Check sheet for the modelled part. Datum: model origin and axes. Units: mm. A direction names the side the tool comes from. Round coordinates to 2 decimals unless told otherwise and drop trailing zeros. Order: outer loops, then holes, each group sorted by start corner. A loop starts at its lowest first (then second) coordinate and runs counter-clockwise, first axis right, second up. Notation, with made-up numbers: M 43.5,25.5 L 98.5,25.5 A13 cw 98.5,49.5 Z; hole C 22.5,25.25 d6. An arc over 180 degrees is marked long. One line per item, written item: value. Start each with the question number.
(1) Thickness scan on L1, parallel to Y at x = 160.02, z = 13.25; L2, parallel to Y at x = 126.5, z = 30.5; L3, parallel to Z at x = 210.5, y = 43.5. Record the ranges inside material, lowest first.
(2) Depth check by flat-ended pin: pin 1 Ø15 at (y, z) = (-131.5, -23) entering from -X; pin 2 Ø3 at (x, y) = (207, -129) entering from -Z; pin 3 Ø1.5 at (y, z) = (-105.5, 18) entering from -X; pin 4 Ø4.5 at (x, y) = (213.5, -122) entering from +Z. Enter the tip coordinate at first touch or a pass-through.
(3) Cross-section at B-B, the plane y = -83.5. Enter the section's corners in (x, z), and give its area (3 significant figures).
(4) Access from +Z, -Z, +X, -X, +Y, -Y to the whole of each face (thin tool, end or side, straight path). Record for faces 1 (the face through (158, 124.617, 25)), 2 (the face through (161, -72, 25.4)), 3 (the face through (215, -124, 28.566)), 4 (the face through (162, -142.672, 5)), 5 (the face through (210, 120, -13.97)).
(5) Release check for a two-part mould opening along Y. For faces 6 (the face through (163, 130.967, 6)), 7 (the face through (122, -139, 55.88)), 8 (the face through (212.547, 116, -21)), 9 (the face through (160, 61, 27.94)) record: released by +Y, released by -Y, zero draft, split by the parting line, or undercut.
(6) Cross-section at D-D, the plane z = -36. Enter the section's corners in (x, y).
(7) Cross-section at A-A, the plane z = 12.5. Enter the section's corners in (x, y) (3 decimals), and give its area (3 significant figures).
(8) Cross-section at C-C, the plane z = -8. Enter the section's corners in (x, y).
from build123d import *

# Parameters (mm, degrees)
SKETCH7_R                = 36.83
SKETCH7_R_2              = 1.905
BOSS_EXTRUDE1_DEPTH      = 6.35
SKETCH8_R                = 36.83
BOSS_EXTRUDE2_DEPTH      = 25.4
BOSS_EXTRUDE2_DEPTH_BACK = 0.000254
SKETCH9_R                = 34.925
CUT_EXTRUDE4_DEPTH       = 25.4
BOSS_EXTRUDE3_DEPTH      = 3.175
BOSS_EXTRUDE4_DEPTH      = 38.1
BOSS_EXTRUDE4_DEPTH_BACK = 40.64
CUT_EXTRUDE5_START       = -20.32
SKETCH12_W               = 34.495809925
SKETCH12_H               = 261.703089784
CUT_EXTRUDE5_DEPTH       = 48.26
SKETCH18_W               = 80.102069995
SKETCH18_H               = 6.35
SKETCH18_W_2             = 84.52860838
BOSS_EXTRUDE7_DEPTH      = 66.04
BOSS_EXTRUDE7_DEPTH_BACK = 55.88
MAIN_ANGLE_DEPTH         = 274.638700862
SKETCH19_W               = 12.7
SKETCH19_H               = 12.7
CUT_EXTRUDE8_DEPTH       = 45.72
SKETCH20_W               = 18.203212612
SKETCH20_H               = 62.726676146
CUT_EXTRUDE9_DEPTH       = 6.35
CUT_EXTRUDE9_TAPER       = 26
SKETCH23_R               = 1.905
CUT_EXTRUDE10_DEPTH      = 56.88
SKETCH24_W               = 16.196066748
SKETCH24_H               = 62.242020171
BOSS_EXTRUDE10_DEPTH     = 3.81


with BuildPart() as part:
    # Sketch7 → Boss-Extrude1 (new body)
    with BuildSketch(Plane.XY):
        with BuildLine():
            Line((117.378076693, -136.321789995), (117.378076693, 124.616910866))
            Line((117.378076693, 124.616910866), (117.378076693, 130.966910866))
            Line((117.378076693, 130.966910866), (187.228076693, 130.966910866))
            ThreePointArc((187.228076693, 130.966910866), (205.188588935, 123.527423108), (212.628076693, 105.566910866))
            Line((212.628076693, 105.566910866), (212.628076693, -117.271789995))
            ThreePointArc((212.628076693, -117.271789995), (205.188588935, -135.232302238), (187.228076693, -142.671789995))
            Line((187.228076693, -142.671789995), (117.378076693, -142.671789995))
            Line((117.378076693, -142.671789995), (117.378076693, -136.321789995))
        make_face()
        with Locations((159.923076693, 61.116910866)):
            Circle(SKETCH7_R, mode=Mode.SUBTRACT)
        with Locations((159.923076693, -72.821789995)):
            Circle(SKETCH7_R, mode=Mode.SUBTRACT)
        with Locations((198.520756421, 117.007578537)):
            Circle(SKETCH7_R_2, mode=Mode.SUBTRACT)
        with Locations((198.520756421, -128.598951794)):
            Circle(SKETCH7_R_2, mode=Mode.SUBTRACT)
    extrude(amount=BOSS_EXTRUDE1_DEPTH)

    # Sketch8 → Boss-Extrude2 (add, two sides)
    with BuildSketch(Plane.XY.offset(2.54)) as boss_extrude2_sk:
        with Locations((160.02, 60.978458264)):
            Circle(SKETCH8_R)
        with Locations((160.02, -72.960242597)):
            Circle(SKETCH8_R)
    extrude(amount=BOSS_EXTRUDE2_DEPTH)
    extrude(boss_extrude2_sk.sketch, amount=-BOSS_EXTRUDE2_DEPTH_BACK)

    # Sketch9 → Cut-Extrude4 (cut)
    with BuildSketch(Plane(origin=(0, 0, 0), x_dir=(-1, 0, 0), z_dir=(0, 0, -1))):
        with Locations((-160.02, 60.978458264)):
            Circle(SKETCH9_R)
        with Locations((-160.02, -72.960242597)):
            Circle(SKETCH9_R)
    extrude(amount=-CUT_EXTRUDE4_DEPTH, mode=Mode.SUBTRACT)

    # Sketch10 → Boss-Extrude3 (add)
    with BuildSketch(Plane.XY.offset(6.35)):
        with BuildLine():
            Line((187.228076693, 130.966910866), (187.228076693, 105.566910866))
            Line((187.228076693, 105.566910866), (212.628076693, 105.566910866))
            ThreePointArc((212.628076693, 105.566910866), (205.188588935, 123.527423108), (187.228076693, 130.966910866))
        make_face()
        with BuildLine():
            Line((212.628076693, -117.271789995), (187.228076693, -117.271789995))
            Line((187.228076693, -117.271789995), (187.228076693, -142.671789995))
            ThreePointArc((187.228076693, -142.671789995), (205.188588935, -135.232302238), (212.628076693, -117.271789995))
        make_face()
    extrude(amount=-BOSS_EXTRUDE3_DEPTH)

    # Sketch11 → Boss-Extrude4 (add, two sides)
    with BuildSketch(Plane(origin=(0, 0, 0), x_dir=(-1, 0, 0), z_dir=(0, 0, -1))) as boss_extrude4_sk:
        with BuildLine():
            Line((-217.892216682, -132.511789995), (-217.892216682, 120.806910866))
            ThreePointArc((-217.892216682, 120.806910866), (-214.916421579, 127.991115763), (-207.732216682, 130.966910866))
            Line((-207.732216682, 130.966910866), (-187.228076693, 130.966910866))
            ThreePointArc((-187.228076693, 130.966910866), (-205.188588935, 123.527423108), (-212.628076693, 105.566910866))
            Line((-212.628076693, 105.566910866), (-212.628076693, -117.271789995))
            ThreePointArc((-212.628076693, -117.271789995), (-205.188588935, -135.232302238), (-187.228076693, -142.671789995))
            Line((-187.228076693, -142.671789995), (-207.732216682, -142.671789995))
            ThreePointArc((-207.732216682, -142.671789995), (-214.916421579, -139.695994892), (-217.892216682, -132.511789995))
        make_face()
    extrude(amount=BOSS_EXTRUDE4_DEPTH)
    extrude(boss_extrude4_sk.sketch, amount=-BOSS_EXTRUDE4_DEPTH_BACK)

    # Sketch12 → Cut-Extrude5 (cut)
    with BuildSketch(Plane.XY.offset(6.35).offset(CUT_EXTRUDE5_START)):
        with Locations((195.299001462, -6.234634026)):
            Rectangle(SKETCH12_W, SKETCH12_H)
    extrude(amount=-CUT_EXTRUDE5_DEPTH, mode=Mode.SUBTRACT)

    # Sketch18 → Boss-Extrude7 (add, two sides)
    with BuildSketch(Plane(origin=(0, 0, 0), x_dir=(-1, 0, 0), z_dir=(0, 0, -1))) as boss_extrude7_sk:
        with Locations((-157.429111691, 127.791910866)):
            Rectangle(SKETCH18_W, SKETCH18_H)
        with Locations((-159.642380883, -139.496789995)):
            Rectangle(SKETCH18_W_2, SKETCH18_H)
    extrude(amount=BOSS_EXTRUDE7_DEPTH)
    extrude(boss_extrude7_sk.sketch, amount=-BOSS_EXTRUDE7_DEPTH_BACK)

    # Sketch16 → main angle (cut, through all)
    with BuildSketch(Plane(origin=(0, 130.966910866, 0), x_dir=(1, 0, 0), z_dir=(0, 1, 0))):
        Polygon((217.892216682, 26.67), (-101.016881875, 82.73406518), (217.892216682, 82.73406518), align=None)
        Polygon((217.892216682, -32.396277701), (47.589100189, -76.347646381), (217.892216682, -67.47666805), align=None)
    extrude(amount=-MAIN_ANGLE_DEPTH, mode=Mode.SUBTRACT)

    # Sketch19 → Cut-Extrude8 (cut)
    with BuildSketch(Plane(origin=(217.892216682, 0, 0), x_dir=(0, 0, -1), z_dir=(1, 0, 0))):
        with Locations((-22.215809399, -123.786574298)):
            Rectangle(SKETCH19_W, SKETCH19_H)
        with Locations((-22.215809399, 114.456910866)):
            Rectangle(SKETCH19_W, SKETCH19_H)
    extrude(amount=-CUT_EXTRUDE8_DEPTH, mode=Mode.SUBTRACT)

    # Sketch20 → Cut-Extrude9 (cut)
    with BuildSketch(Plane(origin=(0, 0, 0), x_dir=(-1, 0, 0), z_dir=(0, 0, -1))):
        with Locations((-159.923076693, -5.934095423)):
            Rectangle(SKETCH20_W, SKETCH20_H)
    extrude(amount=-CUT_EXTRUDE9_DEPTH, taper=CUT_EXTRUDE9_TAPER, mode=Mode.SUBTRACT)

    # Sketch23 → Cut-Extrude10 (cut, through all)
    with BuildSketch(Plane(origin=(0, 0, 0), x_dir=(-1, 0, 0), z_dir=(0, 0, -1))):
        with Locations((-198.520756421, 117.007578537)):
            Circle(SKETCH23_R)
        with Locations((-198.520756421, -128.598951794)):
            Circle(SKETCH23_R)
    extrude(amount=-CUT_EXTRUDE10_DEPTH, mode=Mode.SUBTRACT)

    # Sketch24 → Boss-Extrude10 (add)
    with BuildSketch(Plane(origin=(0, 0, 2.539746), x_dir=(-1, 0, 0), z_dir=(0, 0, -1))):
        with Locations((-160.078035159, -5.897511229)):
            Rectangle(SKETCH24_W, SKETCH24_H)
    extrude(amount=-BOSS_EXTRUDE10_DEPTH)


solid = part.part
Values found:
1. L1: -142.67 to -136.32, -109.79 to -107.89, -38.04 to -36.13, 24.15 to 26.05, 95.9 to 97.81, 124.62 to 130.97
1. L2: -142.67 to -136.32, 124.62 to 130.97
1. L3: 0 to 6.35
2. pin 1: x = 117.38
2. pin 2: z = 0
2. pin 3: x = 141.42
2. pin 4: z = 33.96
3. outline: M 117.38,0 L 124.68,0 L 124.68,6.35 L 117.38,6.35 Z; M 124.73,2.54 L 126.72,2.54 L 126.72,25.4 L 193.32,25.4 L 193.32,2.54 L 195.17,2.54 L 195.17,0 L 212.63,0 L 212.63,-27.6 L 217.89,-26.67 L 217.89,32.4 L 212.63,33.75 L 212.63,6.35 L 195.31,6.35 L 195.31,27.94 L 124.73,27.94 Z
3. area: 744 mm^2
4. face 1: +Z, -X
4. face 2: -Z
4. face 3: +X, -X
4. face 4: +Z, -Z, +X, -X, -Y
4. face 5: -Z, -X
5. face 6: released by +Y
5. face 7: zero draft
5. face 8: undercut
5. face 9: undercut
6. outline: M 117.38,-142.67 L 164.82,-142.67 L 164.82,-136.32 L 117.38,-136.32 Z; M 117.38,124.62 L 164.82,124.62 L 164.82,130.97 L 117.38,130.97 Z
7. outline: M 117.378,-142.672 L 207.732,-142.672 A10.16 ccw 217.892,-132.512 L 217.892,120.807 A10.16 ccw 207.732,130.967 L 117.378,130.967 L 117.378,124.617 L 197.48,124.617 L 197.48,128.806 A25.4 cw 212.628,105.567 L 212.628,-117.272 A25.4 cw 201.907,-138.001 L 201.907,-136.322 L 117.378,-136.322 Z; C 160.02,-72.96 d73.66; C 160.02,60.978 d73.66; hole C 160.02,-72.96 d69.85; hole C 160.02,60.978 d69.85
7. area: 3,550 mm^2
8. outline: M 117.38,-142.67 L 207.73,-142.67 A10.16 ccw 217.89,-132.51 L 217.89,120.81 A10.16 ccw 207.73,130.97 L 117.38,130.97 L 117.38,124.62 L 197.48,124.62 L 197.48,128.81 A25.4 cw 212.63,105.57 L 212.63,-117.27 A25.4 cw 201.91,-138 L 201.91,-136.32 L 117.38,-136.32 Z
